Can you work these out from the model? Positions are in its coordinate system, mm. Face numbers are marked on the shaded views. A direction names the side the tool comes from. Give positions to 0.01 mm unless a question says otherwise; leave off trailing zeros. Loops run counter-clockwise (first coordinate to the right, second up) from the corner with the lowest first, then second, coordinate; pieces in that order, holes last. Notation, with made-up numbers: (25.25, 70) -> (36.25, 70) arc R11 cw to (36.25, 90) -> close; hole circle Ø8 at (32, 11). An arc over 180 degrees is marked (long way). Return JSON: item names as keys, results as strings. Group by question number.
Q1. Will these pins go through, and if not, where does the flat tip stop? pin 1 (8 mm diameter, centred on y = 1, z = 3, fed in from +X); pin 2 (8 mm diameter, centred on y = -15, z = 2, fed in from +X); pin 3 (2 mm diameter, centred on y = -24.5, z = 10.5, fed in from +X).
Q2. Suppose I cut it at A-A, the plane z = 4. Please give me the cut outline in (x, y), and give its area (3 significant figures).
Q3. I need wall thicknesses on line 1 along Y through (x, z) = (217.5, 13.5); line 2 along Y through (x, z) = (161.5, 5); line 3 along X through (y, z) = (-38, 6.75). Which ranges of each line are inside material? Lowest first, please. Write a range as [from, to].
Q4. Which directions (+Z, -Z, +X, -X, +Y, -Y) give clear straight access to the entire face, cutting with the end or side of a thin tool? Please do the marked faces 1, 2 and 3.
Q5. Suppose I cut it at D-D, the plane x = 153. Please give me the cut outline in (y, z), and give its area (3 significant figures).
Q6. Thinking about a two-plate mould opening in X: for the marked faces 4, 5 and 6, which applies, pulls with the +X half, pulls with the -X half, needs draft (parallel to the pull), parting line crosses it, or undercut?
Q7. Suppose I cut it at B-B, the plane x = 75.5. Please give me the cut outline in (y, z).
Q8. Suppose I cut it at C-C, the plane y = -4.5. Please give me the cut outline in (x, z), and give its area (3 significant figures).
```python
from build123d import *

# Parameters (mm, degrees)
PAD_DEPTH    = 15
SKETCH_W     = 36
SKETCH_H     = 30
SKETCH_W_2   = 50
SKETCH_H_2   = 18
POCKET_DEPTH = 15


with BuildPart() as part:
    # Sketch001 → Pad (new body)
    with BuildSketch(Plane.XY):
        Polygon((-5.375519, -14.003706), (36.6356, -30.130264), (137.251264, -21.327534), (268.922544, -106.835863), (284.17016, -96.456116), (243.071506, 21.266001), (0, 0), align=None)
    extrude(amount=PAD_DEPTH)

    # Sketch (on Face9 of Pad) → Pocket (cut)
    with BuildSketch(Plane.XY.offset(15)):
        with Locations((228, -30)):
            Rectangle(SKETCH_W, SKETCH_H)
        with Locations((175, -3)):
            Rectangle(SKETCH_W_2, SKETCH_H_2)
        Polygon((54.668897, -1.428386), (56.362903, -17.247945), (110.287964, -11.228361), (108.593958, 4.591198), align=None)
        Polygon((202.786784, -67.35767), (207.137526, -60.644173), (270.056785, -101.41956), (265.725821, -108.145875), align=None)
        Polygon((156.748499, -37.544555), (177.712625, -51.164592), (182.071037, -44.456072), (161.106911, -30.836035), align=None)
    extrude(amount=-POCKET_DEPTH, mode=Mode.SUBTRACT)


solid = part.part
```
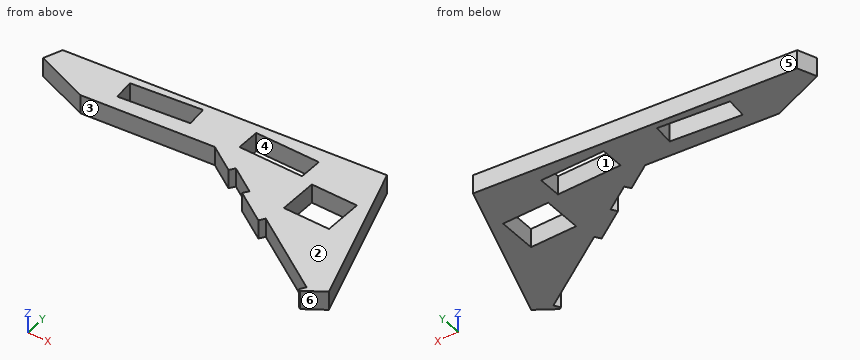
Ans:
{
 "1": {"pin 1": "stops at x = 251.54", "pin 2": "stops at x = 257.13", "pin 3": "stops at x = 259.4"},
 "2": {"outline": "(-5.38, -14) -> (36.64, -30.13) -> (137.25, -21.33) -> (158.37, -35.04) -> (161.11, -30.84) -> (182.07, -44.46) -> (179.34, -48.66) -> (204.37, -64.91) -> (207.14, -60.64) -> (270.06, -101.42) -> (267.26, -105.76) -> (268.92, -106.84) -> (284.17, -96.46) -> (243.07, 21.27) -> (0, 0) -> close; hole (54.67, -1.43) -> (56.36, -17.25) -> (110.29, -11.23) -> (108.59, 4.59) -> close; hole (150, -12) -> (200, -12) -> (200, 6) -> (150, 6) -> close; hole (210, -45) -> (246, -45) -> (246, -15) -> (210, -15) -> close", "area": "11,200 mm^2"},
 "3": {"line 1": "y = [-67.36, -45], [-15, 19.03]", "line 2": "y = [-31.09, -12], [6, 14.13]", "line 3": "x = [172.13, 210], [246, 263.76]"},
 "4": {"face 1": "+Z, -Z", "face 2": "+Z, +X, -X, +Y, -Y", "face 3": "+Z, -Z, -Y"},
 "5": {"outline": "(-31.55, 0) -> (-12, 0) -> (-12, 15) -> (-31.55, 15) -> close; (6, 0) -> (13.39, 0) -> (13.39, 15) -> (6, 15) -> close", "area": "404 mm^2"},
 "6": {"face 4": "undercut", "face 5": "pulls with the -X half", "face 6": "pulls with the +X half"},
 "7": {"outline": "(-26.73, 0) -> (-15.11, 0) -> (-15.11, 15) -> (-26.73, 15) -> close; (0.9, 0) -> (6.61, 0) -> (6.61, 15) -> (0.9, 15) -> close"},
 "8": {"outline": "(-1.73, 0) -> (55, 0) -> (55, 15) -> (-1.73, 15) -> close; (109.57, 0) -> (150, 0) -> (150, 15) -> (109.57, 15) -> close; (200, 0) -> (252.07, 0) -> (252.07, 15) -> (200, 15) -> close", "area": "2,240 mm^2"}
}
